Can you work these out from the model? Positions are in its coordinate system, mm. A direction names the side the tool comes from. Give positions to 0.01 mm unless a question says otherwise; leave off trailing zeros. Order: outer loops, then holes, each group sorted by start corner. A loop starts at its lowest first (then second) coordinate and runs counter-clockwise, first axis right, second up. Notation, with made-up numbers: (18, -26.5) - (44, -26.5) arc R21 cw to (44, -12.5) - close; hole circle Ø8 at (4, 0.25). An arc over 180 degrees is marked (long way). Answer as a JSON object with one key per item and string values.
```python
from build123d import *

# Parameters (mm, degrees)
BASE_DEPTH            = 2
SKETCH3_R             = 7
MOUNTING_BOSSES_DEPTH = 25.4
MOUNTING_BOSSES_TAPER = 6
RIBW_DEPTH            = 5
SKETCH6_R             = 2.286
MOUNTING_HOLES_DEPTH  = 3
SKETCH7_R             = 1.2
SCREW_HOLES_DEPTH     = 26.4


with BuildPart() as part:
    # Sketch2 → Base (new body)
    with BuildSketch(Plane.XY):
        with BuildLine():
            Line((3.808375995, 60.113352729), (87.458375995, 5.873352729))
            ThreePointArc((87.458375995, 5.873352729), (89.523352729, -3.808375995), (79.841624005, -5.873352729))
            Line((79.841624005, -5.873352729), (-3.808375995, 48.366647271))
            ThreePointArc((-3.808375995, 48.366647271), (-5.873352729, 58.048375995), (3.808375995, 60.113352729))
        make_face()
        with BuildLine():
            Line((87.458375995, 48.366647271), (3.808375995, -5.873352729))
            ThreePointArc((3.808375995, -5.873352729), (-5.873352729, -3.808375995), (-3.808375995, 5.873352729))
            Line((-3.808375995, 5.873352729), (79.841624005, 60.113352729))
            ThreePointArc((79.841624005, 60.113352729), (89.523352729, 58.048375995), (87.458375995, 48.366647271))
        make_face()
    extrude(amount=BASE_DEPTH)

    # Sketch3 → Mounting Bosses (add)
    with BuildSketch(Plane.XY):
        with Locations((0, 54.24)):
            Circle(SKETCH3_R)
        Circle(SKETCH3_R)
        with Locations((83.65, 0)):
            Circle(SKETCH3_R)
        with Locations((83.65, 54.24)):
            Circle(SKETCH3_R)
    extrude(amount=MOUNTING_BOSSES_DEPTH, taper=MOUNTING_BOSSES_TAPER)

    # Sketch5 → Ribw (add)
    with BuildSketch(Plane.XY):
        with BuildLine():
            Line((79.841624005, 60.113352729), (41.825, 35.462764731))
            Line((41.825, 35.462764731), (3.808375995, 60.113352729))
            ThreePointArc((3.808375995, 60.113352729), (-5.873352729, 58.048375995), (-3.808375995, 48.366647271))
            Line((-3.808375995, 48.366647271), (28.958623345, 27.12))
            Line((28.958623345, 27.12), (-3.808375995, 5.873352729))
            ThreePointArc((-3.808375995, 5.873352729), (-5.873352729, -3.808375995), (3.808375995, -5.873352729))
            Line((3.808375995, -5.873352729), (41.825, 18.777235269))
            Line((41.825, 18.777235269), (79.841624005, -5.873352729))
            ThreePointArc((79.841624005, -5.873352729), (89.523352729, -3.808375995), (87.458375995, 5.873352729))
            Line((87.458375995, 5.873352729), (54.691376655, 27.12))
            Line((54.691376655, 27.12), (87.458375995, 48.366647271))
            ThreePointArc((87.458375995, 48.366647271), (89.523352729, 58.048375995), (79.841624005, 60.113352729))
        make_face()
        with BuildLine():
            Line((80.494488461, 59.106492261), (42.927832285, 34.747670611))
            Line((42.927832285, 34.747670611), (53.58854437, 27.83509412))
            Line((53.58854437, 27.83509412), (86.805511539, 49.373507739))
            ThreePointArc((86.805511539, 49.373507739), (88.516492261, 57.395511539), (80.494488461, 59.106492261))
        make_face(mode=Mode.SUBTRACT)
        with BuildLine():
            Line((-3.155511539, 49.373507739), (30.06145563, 27.83509412))
            Line((30.06145563, 27.83509412), (40.722167715, 34.747670611))
            Line((40.722167715, 34.747670611), (3.155511539, 59.106492261))
            ThreePointArc((3.155511539, 59.106492261), (-4.866492261, 57.395511539), (-3.155511539, 49.373507739))
        make_face(mode=Mode.SUBTRACT)
        with BuildLine():
            Line((30.06145563, 26.40490588), (40.722167715, 19.492329389))
            Line((40.722167715, 19.492329389), (3.155511539, -4.866492261))
            ThreePointArc((3.155511539, -4.866492261), (-4.866492261, -3.155511539), (-3.155511539, 4.866492261))
            Line((-3.155511539, 4.866492261), (30.06145563, 26.40490588))
        make_face(mode=Mode.SUBTRACT)
        Polygon((31.164287915, 27.12), (41.825, 20.207423508), (52.485712085, 27.12), (41.825, 34.032576492), align=None, mode=Mode.SUBTRACT)
        with BuildLine():
            Line((42.927832285, 19.492329389), (80.494488461, -4.866492261))
            ThreePointArc((80.494488461, -4.866492261), (88.516492261, -3.155511539), (86.805511539, 4.866492261))
            Line((86.805511539, 4.866492261), (53.58854437, 26.40490588))
            Line((53.58854437, 26.40490588), (42.927832285, 19.492329389))
        make_face(mode=Mode.SUBTRACT)
    extrude(amount=RIBW_DEPTH)

    # Sketch6 → Mounting Holes (cut, through all)
    with BuildSketch(Plane.XY.offset(2)):
        with Locations((10.563469491, 6.849522835)):
            Circle(SKETCH6_R)
        with Locations((10.563469491, 47.390477165)):
            Circle(SKETCH6_R)
        with Locations((73.351093758, 47.562024213)):
            Circle(SKETCH6_R)
        with Locations((73.086530509, 6.849522835)):
            Circle(SKETCH6_R)
    extrude(amount=-MOUNTING_HOLES_DEPTH, mode=Mode.SUBTRACT)

    # Sketch7 → Screw Holes (cut, through all)
    with BuildSketch(Plane.XY.offset(25.4)):
        Circle(SKETCH7_R)
        with Locations((0, 54.24)):
            Circle(SKETCH7_R)
        with Locations((83.65, 54.24)):
            Circle(SKETCH7_R)
        with Locations((83.65, 0)):
            Circle(SKETCH7_R)
    extrude(amount=-SCREW_HOLES_DEPTH, mode=Mode.SUBTRACT)


solid = part.part
```
Q1. Which directions (+Z, -Z, +X, -X, +Y, -Y) give clear straight access to the entire face, cutting with the end or side of a thin tool? Please do faces 5 (the face through (69.206, 16.279, 3.479)), 6 (the face through (89.438, 58.177, 2.465)).
Recorded:
{"face 5": "+Z", "face 6": "+Z, -Z"}
Q2. If we section it at A-A, the plane z = 22.75: Please give me the cut outline in (x, y), then the cut area to 3 significant figures.
Recorded:
{"outline": "circle Ø9.22 at (0, 0); circle Ø9.22 at (0, 54.24); circle Ø9.22 at (83.65, 0); circle Ø9.22 at (83.65, 54.24); hole circle Ø2.4 at (0, 0); hole circle Ø2.4 at (0, 54.24); hole circle Ø2.4 at (83.65, 0); hole circle Ø2.4 at (83.65, 54.24)", "area": "249 mm^2"}
Q3. If we section it at D-D, the plane x = 65: Please give me the cut outline in (y, z).
Recorded:
{"outline": "(3.75, 0) - (20.44, 0) - (20.44, 5) - (19.01, 5) - (19.01, 2) - (5.18, 2) - (5.18, 5) - (3.75, 5) - close; (33.8, 0) - (50.49, 0) - (50.49, 5) - (49.06, 5) - (49.06, 2) - (35.23, 2) - (35.23, 5) - (33.8, 5) - close"}
Q4. If we section it at B-B, the plane y = 42: Please give me the cut outline in (x, z), then the cut area to 3 significant figures.
Recorded:
{"outline": "(6.01, 0) - (31.74, 0) - (31.74, 5) - (29.54, 5) - (29.54, 2) - (8.22, 2) - (8.22, 5) - (6.01, 5) - close; (51.91, 0) - (77.64, 0) - (77.64, 5) - (75.43, 5) - (75.43, 2) - (54.11, 2) - (54.11, 5) - (51.91, 5) - close", "area": "129 mm^2"}
Q5. I need wall thicknesses on L1, parallel to Y at x = 59, z = 4.5; L2, parallel to Y at x = 0, z = 5.25; L3, parallel to X at y = 5, z = 3.5. Which ranges of each line are inside material? Lowest first, please.
Recorded:
{"L1": "y = 7.64 to 9.07, 22.9 to 24.33, 29.91 to 31.34, 45.17 to 46.6", "L2": "y = -6.45 to -1.2, 1.2 to 6.45, 47.79 to 53.04, 55.44 to 60.69", "L3": "x = -4.9 to 4.36, 18.37 to 20.58, 63.07 to 65.28, 79.29 to 88.55"}
Q6. I'm going to push flat-ended pins straight in: pin 1 Ø12 at (x, z) = (77.5, 15.5) entering from +Y; pin 2 Ø2 at (x, y) = (0, 0) entering from -Z; pin 3 Ø23.5 at (x, y) = (66.5, 9) entering from +Z; pin 4 Ø8 at (x, y) = (71.5, 8.5) entering from +Z. Where does each tip first touch, or does it pass through?
Recorded:
{"pin 1": "stops at y = 59.85", "pin 2": "passes through", "pin 3": "stops at z = 5", "pin 4": "stops at z = 2"}
Q7. We'd pull the mould along Y, two halves only. Please class faces 1 (the face through (36.42, 23.71, 3.48)), 2 (the face through (1, 53, 25.4)), 3 (the face through (61.1, 6.28, 2.46)), 4 (the face through (23, 8, 3)): released by +Y, released by -Y, zero draft, split by the parting line, or undercut.
Recorded:
{"face 1": "undercut", "face 2": "zero draft", "face 3": "released by -Y", "face 4": "undercut"}
Q8. If we section it at C-C, the plane x = 10: Please give me the cut outline in (y, z) (3 decimals), then the cut area to 3 significant figures.
Recorded:
{"outline": "(-1.859, 0) - (4.634, 0) - (4.634, 2) - (-0.428, 2) - (-0.428, 5) - (-1.859, 5) - close; (9.065, 0) - (14.827, 0) - (14.827, 5) - (13.397, 5) - (13.397, 2) - (9.065, 2) - close; (39.413, 0) - (45.175, 0) - (45.175, 2) - (40.843, 2) - (40.843, 5) - (39.413, 5) - close; (49.606, 0) - (56.099, 0) - (56.099, 5) - (54.668, 5) - (54.668, 2) - (49.606, 2) - close", "area": "66.2 mm^2"}
